Verification items for the finished model (mm, model axes). Round coordinates to 2 decimals unless told otherwise and drop trailing zeros. Write each loop counter-clockwise with the first axis right and the second up, starting at its lowest first coordinate (ties: lowest second). Pieces come first, ordered by that corner, then holes. Notation, with made-up numbers: M 50.25,-27 L 70.25,-27 A16 cw 70.25,-4 Z; hole C 89,6.25 d4. An arc over 180 degrees is marked long. Answer in a Markdown table with one row per item. Add a question column.
1. Material ranges on probe 1 along X at (y, z) = (-1.5, 26.5); probe 2 along Y at (x, z) = (-24, 62); probe 3 along Y at (x, z) = (-18, 9), recorded low to high.
2. Go/stop test with flat-tipped pins: pin 1 Ø2 at (y, z) = (-26.5, 11) entering from -X; pin 2 Ø3 at (y, z) = (9.5, 34) entering from -X; pin 3 Ø2 at (x, z) = (-2.5, 48.5) entering from -Y. Record where each tip stops, or that it passes through.
3. Sectioned sample at A-A on z = 31. Record the cut outline in (x, y), plus the area to 3 significant figures.
```python
from build123d import *

# Parameters (mm, degrees)
F0_R     = 34.385089
F1_DEPTH = 68.834
F2_R     = 5.08
F3_R     = 5.08


with BuildPart() as f1:
    # F0 (on Top) → F1 (new body)
    with BuildSketch(Plane.XY):
        Circle(F0_R)
    extrude(amount=F1_DEPTH)

    # F2
    f2_edges = [f1.edges().sort_by_distance(p)[0] for p in [
        (-34.385089, 0, 68.834),
    ]]
    fillet(f2_edges, radius=F2_R)

    # F3
    f3_edges = [f1.edges().sort_by_distance(p)[0] for p in [
        (34.385089, 0, 31.877),
        (-34.385089, 0, 63.754),
        (-34.385089, 0, 0),
    ]]
    fillet(f3_edges, radius=F3_R)


solid = f1.part
```
Geometry check:
| question | item | result |
|---|---|---|
| 1 | probe 1 | x = -34.35 to 34.35 |
| 1 | probe 2 | y = -24.62 to 24.62 |
| 1 | probe 3 | y = -29.3 to 29.3 |
| 2 | pin 1 | stops at x = -23.07 |
| 2 | pin 2 | stops at x = -33.44 |
| 2 | pin 3 | stops at y = -34.35 |
| 3 | outline | C 0,0 d68.77 |
| 3 | area | 3,710 mm2 |
